Work out the finished part from the listing and answer in its coordinate system (mm). Round coordinates to 2 decimals unless told otherwise and drop trailing zeros. Order: outer loops, then holes, each group sorted by start corner. A loop starts at its lowest first (then second) coordinate and runs counter-clockwise, first axis right, second up. Notation, with made-up numbers: M -37,10.25 L -17,10.25 A16 ccw -17,22.25 Z; hole C 73,67.25 d7. An arc over 180 degrees is marked long. Answer as a JSON object with one key per item and string values. Group by question number.
from build123d import *

# Parameters (mm, degrees)
SKETCH1_R           = 21
BOSS_EXTRUDE1_DEPTH = 15
FILLET1_R           = 1
SKETCH2_R           = 4.5
CUT_EXTRUDE1_DEPTH  = 15


with BuildPart() as part:
    # Sketch1 → Boss-Extrude1 (new body)
    with BuildSketch(Plane(origin=(0, 0, 0), x_dir=(0, 0, -1), z_dir=(1, 0, 0))):
        Circle(SKETCH1_R)
    extrude(amount=-BOSS_EXTRUDE1_DEPTH)

    # Fillet1
    fillet1_edges = [part.edges().sort_by_distance(p)[0] for p in [
        (0, 0, 21),
        (-15, 0, 21),
    ]]
    fillet(fillet1_edges, radius=FILLET1_R)

    # Sketch2 → Cut-Extrude1 (cut)
    with BuildSketch(Plane(origin=(0, 0, 0), x_dir=(0, 0, -1), z_dir=(1, 0, 0))):
        Circle(SKETCH2_R)
    extrude(amount=-CUT_EXTRUDE1_DEPTH, mode=Mode.SUBTRACT)


solid = part.part
Item 1: The mould has two halves that part along Y. Classify faces 1 (the cylindrical face through (-7.41, 6.31, -20.03)), 2 (the flat face through (-15, 5, 0)), 3 (the cylindrical face through (-7.4, 4.46, 0.59)): +Y half, -Y half, draft (parallel to the pull), parting line (faces both ways), or undercut.
Item 2: Find section A-A (y = 0). Give the vertices of the cut face in (x, z), and give its area (3 significant figures).
Item 3: Find section B-B (x = -4.5). Give the vertices of the cut face in (y, z).
Item 4: Consider L1, parallel to Y at x = -9.75, z = 0; L2, parallel to X at y = -18.5, z = 8; L3, parallel to Y at x = -13, z = -5. Determine where each line is inside the solid, lowest interval first.
Item 5: Each of these flat-tipped pins is pushed along its axis until it touches: pin 1 (8 mm diameter, centred on x = -10.5, z = 2.5, fed in from +Y); pin 2 (2 mm diameter, centred on x = -8, y = 13.5, fed in from +Z); pin 3 (4 mm diameter, centred on x = -2.5, z = 10.5, fed in from -Y). Where does it stop, or does it pass through?
Responses:
{
 "1": {"face 1": "parting line", "face 2": "draft", "face 3": "undercut"},
 "2": {"outline": "M -15,-20 A1 ccw -14,-21 L -1,-21 A1 ccw 0,-20 L 0,-4.5 L -15,-4.5 Z; M -15,4.5 L 0,4.5 L 0,20 A1 ccw -1,21 L -14,21 A1 ccw -15,20 Z", "area": "494 mm^2"},
 "3": {"outline": "C 0,0 d42; hole C 0,0 d9"},
 "4": {"L1": "y = -21 to -4.5, 4.5 to 21", "L2": "x = -14.99 to -0.01", "L3": "y = -20.4 to 20.4"},
 "5": {"pin 1": "stops at y = 21", "pin 2": "stops at z = 16.87", "pin 3": "stops at y = -19.2"}
}
